Build history of the part. All positions in model axes, mm. A direction names the side the tool comes from. Round coordinates to 2 decimals unless told otherwise and drop trailing zeros. Loops run counter-clockwise (first coordinate to the right, second up) from the corner with the lowest first, then second, coordinate; pieces in that order, holes last.
from build123d import *

# Parameters (mm, degrees)
F0_R     = 54.2373260285
F1_DEPTH = 12.7
F3_START = 54.6908248216
F2_R     = 15.7906260278
F3_DEPTH = 89.0027470887


with BuildPart() as f1:
    # F0 (on Top) → F1 (new body)
    with BuildSketch(Plane.XY):
        with BuildLine():
            ThreePointArc((5.5742384489, -21.0680376267), (45.7140278431, -1.1655540145), (61.9223292112, 40.6028851867))
            ThreePointArc((61.9223292112, 40.6028851867), (60.33472157, 54.5347274197), (55.653307019, 67.7521811772))
            ThreePointArc((55.653307019, 67.7521811772), (48.7942433887, 78.7276365572), (39.8035687607, 88.0375852368))
            ThreePointArc((39.8035687607, 88.0375852368), (26.5437780286, 96.5475248129), (11.5655175366, 101.4355545268))
            ThreePointArc((11.5655175366, 101.4355545268), (-0.9231515567, 102.5183327433), (-13.3739883144, 101.0637096229))
            ThreePointArc((-13.3739883144, 101.0637096229), (-27.3748629814, 96.1455870627), (-39.8035687607, 88.0375852368))
            ThreePointArc((-39.8035687607, 88.0375852368), (-48.7942433887, 78.7276365572), (-55.653307019, 67.7521811772))
            ThreePointArc((-55.653307019, 67.7521811772), (-53.9394187779, 10.190487109), (-5.5742384489, -21.0680376267))
            Line((-5.5742384489, -21.0680376267), (5.5742384489, -21.0680376267))
        make_face()
        with Locations((0, 40.6028851867)):
            Circle(F0_R, mode=Mode.SUBTRACT)
        with BuildLine():
            ThreePointArc((-13.3739883144, 101.0637096229), (-0.9231515567, 102.5183327433), (11.5655175366, 101.4355545268))
            Line((11.5655175366, 101.4355545268), (0, 138.1439715624))
            Line((0, 138.1439715624), (-13.3739883144, 101.0637096229))
        make_face()
        with BuildLine():
            ThreePointArc((39.8035687607, 88.0375852368), (48.7942433887, 78.7276365572), (55.653307019, 67.7521811772))
            Line((55.653307019, 67.7521811772), (65.5085667968, 101.0637096229))
            Line((65.5085667968, 101.0637096229), (39.8035687607, 88.0375852368))
        make_face()
        with BuildLine():
            Line((5.6826770306, -21.0680376267), (5.5742384489, -21.0680376267))
            ThreePointArc((5.5742384489, -21.0680376267), (0, -21.3194440245), (-5.5742384489, -21.0680376267))
            Line((-5.5742384489, -21.0680376267), (-5.5742384489, -58.2595206797))
            Line((-5.5742384489, -58.2595206797), (5.6826770306, -58.2595206797))
            Line((5.6826770306, -58.2595206797), (5.6826770306, -21.0680376267))
        make_face()
        with BuildLine():
            ThreePointArc((-5.5742384489, -21.0680376267), (0, -21.3194440245), (5.5742384489, -21.0680376267))
            Line((5.5742384489, -21.0680376267), (-5.5742384489, -21.0680376267))
        make_face()
        with BuildLine():
            Line((-63.6594295502, 101.0637096229), (-55.653307019, 67.7521811772))
            ThreePointArc((-55.653307019, 67.7521811772), (-48.7942433887, 78.7276365572), (-39.8035687607, 88.0375852368))
            Line((-39.8035687607, 88.0375852368), (-63.6594295502, 101.0637096229))
        make_face()
        Polygon((5.6826770306, -58.2595206797), (-5.5742384489, -58.2595206797), (-13.3375748992, -58.2595206797), (-13.3375748992, -143.073156476), (13.1347030401, -143.073156476), (13.1347030401, -58.2595206797), align=None)
    extrude(amount=F1_DEPTH)

    # F2 (on Front) → F3 (join)
    with BuildSketch(Plane.XZ.offset(F3_START)):
        with Locations((0, 6.2494464219)):
            Circle(F2_R)
    extrude(amount=F3_DEPTH)


solid = f1.part
(1) Which spindle directions (+Z, -Z, +X, -X, +Y, -Y) get a long thin tool onto all of the face, cutting with end or side? Do faces 1 (the face through (20, 92, 12.7)), 2 (the face through (5.683, -38, 6)), 3 (the face through (52.836, 94.642, 6.261)). Say none if no direction does.
Responses:
face 1: +Z, +X, -X, +Y
face 2: +Z, -Z, +X
face 3: +Z, -Z, +Y
(2) Pull direction X, two halves, no side cores. Call faces 4 (the face through (26.743, 96.452, 6.261)), 5 (the face through (-27.188, 96.237, 6.261)), 6 (the face through (7.286, -98.569, -7.76)), 7 (the face through (-6.593, 119.863, 6.261)): +X half, -X half, draft (parallel to the pull), parting line (faces both ways), or undercut.
Responses:
face 4: undercut
face 5: undercut
face 6: parting line
face 7: -X half
(3) Probe line 1 (X direction, y = 97.5, z = 8.5); line 2 (Y direction, x = -15, z = 5); line 3 (X direction, y = 55.5, z = 4). List the from-to ranges inside material, lowest first.
Responses:
line 1: x = -62.8 to -57.13, -24.44 to 24.44, 58.48 to 64.45
line 2: y = -143.69 to -54.69, -19.48 to -11.52, 92.72 to 100.68
line 3: x = -60.1 to -52.15, 52.15 to 60.1
(4) Slice it at A-A on y = 23. List the corners of the cut face in (x, z), plus the area to 3 significant figures.
Responses:
outline: (-59.37, 0) - (-51.3, 0) - (-51.3, 12.7) - (-59.37, 12.7) - close; (51.3, 0) - (59.37, 0) - (59.37, 12.7) - (51.3, 12.7) - close
area: 205 mm2
(5) Slice it at B-B on x = 50. List the corners of the cut face in (y, z), plus the area to 3 significant figures.
Responses:
outline: (4.07, 0) - (19.59, 0) - (19.59, 12.7) - (4.07, 12.7) - close; (61.62, 0) - (93.2, 0) - (93.2, 12.7) - (61.62, 12.7) - close
area: 598 mm2
(6) Slice it at D-D on z = 18. List the corners of the cut face in (x, y), plus the area to 3 significant figures.
Responses:
outline: (-10.55, -143.69) - (10.55, -143.69) - (10.55, -54.69) - (-10.55, -54.69) - close
area: 1,880 mm2
(7) Slice it at C-C on y = -38. List the corners of the cut face in (x, z), plus the area to 3 significant figures.
Responses:
outline: (-5.57, 0) - (5.68, 0) - (5.68, 12.7) - (-5.57, 12.7) - close
area: 143 mm2
(8) Pin check, flat tips, straight feed: P1, Ø4, axis at y = -32, z = 4.5, coming from the +X side; P2, Ø1.5, axis at y = 96.5, z = 4.5, coming from the -X side; P3, Ø10, axis at y = -75.5, z = 7, coming from the +X side. Stop position of each tip, or through.
Responses:
P1: stops at x = 5.68
P2: stops at x = -62.74
P3: stops at x = 15.79
